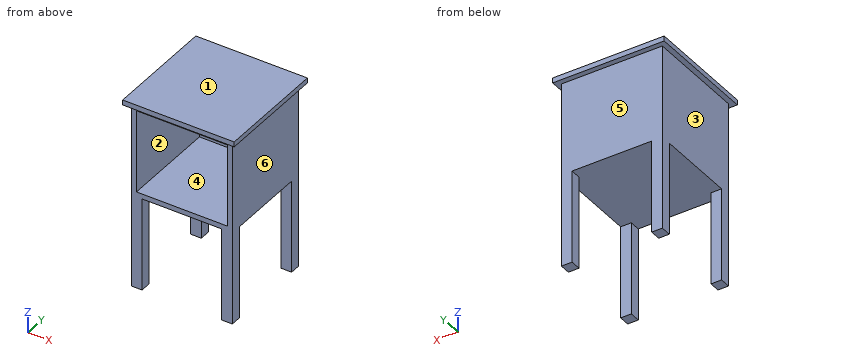
```python
from build123d import *

# Parameters (mm, degrees)
F0_W      = 380
F0_H      = 380
F1_DEPTH  = 350
F2_W      = 342
F2_H      = 312
F3_DEPTH  = 361
F4_W      = 342
F4_H      = 312
F5_DEPTH  = 361
F6_W      = 40
F6_H      = 40
F7_DEPTH  = 150
F8_W      = 40
F8_H      = 40
F9_DEPTH  = 150
F10_W     = 40
F10_H     = 40
F11_DEPTH = 150
F12_W     = 40
F12_H     = 40
F13_DEPTH = 150
F14_W     = 420
F14_H     = 420
F14_W_2   = 380
F14_H_2   = 380
F15_DEPTH = 19
F16_DEPTH = 200


with BuildPart() as f1:
    # F0 (on Top) → F1 (new body)
    with BuildSketch(Plane.XY):
        Rectangle(F0_W, F0_H)
    extrude(amount=F1_DEPTH)

    # F2 (on face) → F3 (join)
    with BuildSketch(Plane.XZ.offset(190)):
        with Locations((0, 175)):
            Rectangle(F2_W, F2_H)
    extrude(amount=-F3_DEPTH)

    # F4 (on face) → F5 (cut)
    with BuildSketch(Plane.XZ.offset(190)):
        with Locations((0, 175)):
            Rectangle(F4_W, F4_H)
    extrude(amount=-F5_DEPTH, mode=Mode.SUBTRACT)

    # F6 (on face) → F7 (join)
    with BuildSketch(Plane(origin=(0, 0, 0), x_dir=(1, 0, 0), z_dir=(0, 0, -1))):
        with Locations((-170, 170)):
            Rectangle(F6_W, F6_H)
    extrude(amount=F7_DEPTH)

    # F8 (on face) → F9 (join)
    with BuildSketch(Plane(origin=(0, 0, 0), x_dir=(1, 0, 0), z_dir=(0, 0, -1))):
        with Locations((170, 170)):
            Rectangle(F8_W, F8_H)
    extrude(amount=F9_DEPTH)

    # F10 (on face) → F11 (join)
    with BuildSketch(Plane(origin=(0, 0, 0), x_dir=(1, 0, 0), z_dir=(0, 0, -1))):
        with Locations((-170, -170)):
            Rectangle(F10_W, F10_H)
    extrude(amount=F11_DEPTH)

    # F12 (on face) → F13 (join)
    with BuildSketch(Plane(origin=(0, 0, 0), x_dir=(1, 0, 0), z_dir=(0, 0, -1))):
        with Locations((170, -170)):
            Rectangle(F12_W, F12_H)
    extrude(amount=F13_DEPTH)

    # F14 (on face) → F15 (join)
    with BuildSketch(Plane.XY.offset(350)):
        Rectangle(F14_W, F14_H)
        Rectangle(F14_W_2, F14_H_2, mode=Mode.SUBTRACT)
        Rectangle(F14_W_2, F14_H_2)
    extrude(amount=F15_DEPTH)

    # F16 (add): faces of the model
    f16_faces = [f1.faces().sort_by_distance(p)[0] for p in [
        (-170, -170, -150),
        (170, -170, -150),
        (-170, 170, -150),
        (170, 170, -150),
    ]]
    extrude(f16_faces, amount=F16_DEPTH)


solid = f1.part
```
Part model, mm, in its own coordinate system. Face numbers are marked on the shaded views. A direction names the side the tool comes from. Round coordinates to 2 decimals unless told otherwise and drop trailing zeros. Loops run counter-clockwise (first coordinate to the right, second up) from the corner with the lowest first, then second, coordinate; pieces in that order, holes last.
1. 3-axis set-ups, long thin cutter, end or side, ignore diameter. For the marked faces 5 and 6: which of +Z, -Z, +X, -X, +Y, -Y reach the whole face in a straight line?
Solutions:
face 5: -Z, +X, -X, +Y
face 6: -Z, +X, +Y, -Y
2. Slice it at C-C (y = 139). Give the cut face in (x, z).
Solutions:
outline: (-210, 350) - (-190, 350) - (-190, 0) - (190, 0) - (190, 350) - (210, 350) - (210, 369) - (-210, 369) - close; hole (-171, 19) - (171, 19) - (171, 331) - (-171, 331) - close
3. Slice it at B-B (x = 29). Give the cut face in (y, z), and give its area (3 significant figures).
Solutions:
outline: (-210, 350) - (-190, 350) - (-190, 331) - (171, 331) - (171, 19) - (-190, 19) - (-190, 0) - (190, 0) - (190, 350) - (210, 350) - (210, 369) - (-210, 369) - close
area: 28,300 mm2
4. Flat gauge pins, fed straight in: pin 1 (1 mm diameter, centred on x = 61.5, z = 98, fed in from -Y); pin 2 (20 mm diameter, centred on y = 176.5, z = -191.5, fed in from +X); pin 3 (12 mm diameter, centred on y = 170, z = -91, fed in from -X). Where does each tip first touch, or does it go through?
Solutions:
pin 1: stops at y = 171
pin 2: stops at x = 190
pin 3: stops at x = -190
5. Slice it at D-D (z = 151). Give the cut face in (x, y).
Solutions:
outline: (-190, -190) - (-171, -190) - (-171, 171) - (171, 171) - (171, -190) - (190, -190) - (190, 190) - (-190, 190) - close
6. Two-plate mould, pull along Z, no slides. Class the marked faces 1, 2, 3 and 4: pulls with the +Z half, pulls with the -Z half, needs draft (parallel to the pull), parting line crosses it, or undercut.
Solutions:
face 1: pulls with the +Z half
face 2: undercut
face 3: needs draft
face 4: undercut
7. Drill centre lines: line 1 along X through (y, z) = (-101, 43); line 2 along Z through (x, y) = (168, 149); line 3 along X through (y, z) = (-185.5, -281). Where is each one in solid material? Low to high.
Solutions:
line 1: x = -190 to -171, 171 to 190
line 2: z = 0 to 19, 331 to 369
line 3: x = -190 to -150, 150 to 190
8. Slice it at A-A (z = -55). Give the cut face in (x, y).
Solutions:
outline: (-190, -190) - (-150, -190) - (-150, -150) - (-190, -150) - close; (-190, 150) - (-150, 150) - (-150, 190) - (-190, 190) - close; (150, -190) - (190, -190) - (190, -150) - (150, -150) - close; (150, 150) - (190, 150) - (190, 190) - (150, 190) - close
